Autodesk Inventor part; units mm, degrees
ref_plane "YZ Plane" through (0, 0, 0) normal (1, 0, 0) x (0, 1, 0)
ref_plane "XZ Plane" through (0, 0, 0) normal (0, 1, 0) x (-1, 0, 0)
ref_plane "XY Plane" through (0, 0, 0) normal (0, 0, 1) x (1, 0, 0)
sketch "Sketch1" plane through (0, 0, 0) normal (1, 0, 0) x (0, 1, 0)
  circle A0 centre (0, 0) radius 11
  circle A1 centre (0, 0) radius 22
  circle A2 centre (0, 0) radius 17.5
  circle A3 centre (17.5, 0) radius 2.75
  circle A4 centre (-8.75, 15.1554) radius 2.75
  circle A5 centre (-8.75, -15.1554) radius 2.75
  dimension "d2" = 35
  dimension "d0" = 22
  dimension "d1" = 44
  dimension "d3" = 5.5
  dimension "d6" = 360
extrude "Extrusion1" add sketch "Sketch1" along normal blind 7.5 contours A1 | A3 A2 A5 A4
sketch "Sketch2" plane through (7.5, 0, 0) normal (1, 0, 0) x (0, 0, -1)
  arc A0 (2.7415, 17.2839) -> (-2.7415, 17.2839) centre (0, 0) ccw
  circle A1 centre (0, 0) radius 17.5
  circle A2 centre (0, 17.5) radius 2.75
  circle A3 centre (-15.1554, -8.75) radius 2.75
  circle A4 centre (15.1554, -8.75) radius 2.75
  dimension "d10" = 35
  dimension "d11" = 5.5
  dimension "d14" = 360
extrude "Extrusion2" cut sketch "Sketch2" against normal blind 10 contours A2 A0 | A0 A2 | A3 A1 | A1 A3 | A4 A1 | A1 A4
sketch "Sketch3" plane through (7.5, 0, 0) normal (1, 0, 0) x (0, 0, -1)
  line L0 (0, 0) -> (0, -25)
  line L1 (0, 0) -> (25, 0) construction
  line L2 (0, -25) -> (50, -25)
  line L3 (0, -25) -> (25, -25)
  line L4 (25, -25) -> (25, -20)
  line L5 (25, -20) -> (0, -20)
  line L6 (0, -20) -> (0, -25)
  line L7 (0, -20) -> (30, -20)
  line L8 (30, -20) -> (30, -25)
  line L9 (30, -25) -> (0, -25)
  line L10 (0, -25) -> (0, -20)
  line L11 (30, -25) -> (-30, -25)
  line L12 (-30, -25) -> (-30, -20)
  line L13 (-30, -20) -> (30, -20)
  line L14 (30, -20) -> (30, -25)
  circle A0 centre (0, 0) radius 22
  line L15 (25, -25) -> (-22, -25)
  line L16 (-22, -25) -> (-22, 0)
  line L17 (-22, 0) -> (25, 0)
  line L18 (22, 0) -> (-22, 0)
  line L19 (-22, 0) -> (-22, -25)
  line L20 (-22, -25) -> (22, -25)
  line L21 (22, -25) -> (22, 0)
  line L22 (30, -20) -> (22, -20)
  line L23 (22, -20) -> (22, -25)
  line L24 (22, -25) -> (30, -25)
  line L25 (30, -25) -> (30, -20)
  line L26 (-30, -20) -> (-22, -20)
  line L27 (-22, -20) -> (-22, -25)
  line L28 (-22, -25) -> (-30, -25)
  line L29 (-30, -25) -> (-30, -20)
  dimension "d18" = 25
  dimension "d19" = 90
  dimension "d20" = 50
  dimension "d21" = 25
  dimension "d22" = 5
  dimension "d23" = 30
  dimension "d24" = 5
  dimension "d25" = 60
  dimension "d26" = 5
extrude "Extrusion3" add sketch "Sketch3" against normal blind 7.5 contours L5 A0 L0 | A0 L13 L16 | L21 L5 A0 | A0 L5 L21 L2 L0 | L0 L11 L16 L13 A0 | L16 L11 L12 L13 | L5 L4 L2 L21 | L7 L8 L2 L4
sketch "Sketch5" plane through (7.5, 0, 0) normal (1, 0, 0) x (0, 0, -1)
  line L0 (30, -20) -> (30, -25)
  line L1 (22, -20) -> (30, -20)
  line L2 (30, -25) -> (22, -25)
  line L3 (22, -25) -> (22, -20)
  line L4 (22, -20) -> (30, -20)
  line L5 (30, -20) -> (30, -25)
  line L6 (-30, -20) -> (-30, -25)
  line L7 (-30, -25) -> (-22, -25)
  line L8 (-22, -25) -> (-22, -20)
  line L9 (-22, -20) -> (-30, -20)
  line L10 (-30, -20) -> (-30, -25)
  point P0 (0, 0)
extrude "Extrusion5" add sketch "Sketch5" along normal blind 5
sketch "Sketch8" plane through (0, -20, 30) normal (0, 1, 0) x (1, 0, 0)
  circle A0 centre (3.125, 4) radius 1.5
  circle A1 centre (9.375, 4) radius 1.5
  circle A2 centre (9.375, 56) radius 1.5
  circle A3 centre (3.125, 56) radius 1.5
  point P0 (0, 8)
  point P1 (12.5, 0)
  point P2 (12.5, 52)
  point P3 (0, 60)
  point P4 (0, 52)
extrude "Extrusion7" cut sketch "Sketch8" against normal blind 5
properties part number "Slipring_mount"
Part model, mm, in its own coordinate system. A direction names the side the tool comes from. Give positions to 0.01 mm unless a question says otherwise; leave off trailing zeros. Loops run counter-clockwise (first coordinate to the right, second up) from the corner with the lowest first, then second, coordinate; pieces in that order, holes last. Notation, with made-up numbers: M -4.5,68.5 L 21.5,68.5 A12 cw 21.5,83.5 Z; hole C -5,77 d11. An arc over 180 degrees is marked long. Return JSON: item names as keys, results as strings.
1) Drill centre lines: line 1 (X direction, y = -21.65, z = -26) (3 decimals); line 2 (Z direction, x = 3.5, y = 0); line 3 (Z direction, x = 3.25, y = -7). Where is each one in solid material? Low to high.
Calculated:
{"line 1": "x = 0 to 1.625, 4.625 to 7.875, 10.875 to 12.5", "line 2": "z = -22 to -11, 11 to 22", "line 3": "z = -22 to -17.28, -13.03 to -8.49, 8.49 to 13.03, 17.28 to 22"}
2) Saw through at C-C, the plane x = 5.75. List the corners of the cut face in (y, z), then the cut area to 3 significant figures.
Calculated:
{"outline": "M -25,-30 L -20,-30 L -20,-22 L 0,-22 A22 ccw 0,22 L -20,22 L -20,30 L -25,30 Z; hole C -8.75,-15.16 d5.5; hole C -8.75,15.16 d5.5; hole C 0,0 d22; hole C 17.5,0 d5.5", "area": "1,490 mm2"}
3) Saw through at B-B, the plane y = -8.75. List the corners of the cut face in (x, z).
Calculated:
{"outline": "M 0,-22 L 7.5,-22 L 7.5,-17.91 L 0,-17.91 Z; M 0,-12.41 L 7.5,-12.41 L 7.5,-6.67 L 0,-6.67 Z; M 0,6.67 L 7.5,6.67 L 7.5,12.41 L 0,12.41 Z; M 0,17.91 L 7.5,17.91 L 7.5,22 L 0,22 Z"}
4) Saw through at D-D, the plane x = 3. List the corners of the cut face in (y, z), then the cut area to 3 significant figures.
Calculated:
{"outline": "M -25,-30 L -20,-30 L -20,-27.49 L -25,-27.49 Z; M -25,-24.51 L -20,-24.51 L -20,-22 L 0,-22 A22 ccw 0,22 L -20,22 L -20,24.51 L -25,24.51 Z; M -25,27.49 L -20,27.49 L -20,30 L -25,30 Z; hole C -8.75,-15.16 d5.5; hole C -8.75,15.16 d5.5; hole C 0,0 d22; hole C 17.5,0 d5.5", "area": "1,460 mm2"}
5) Saw through at A-A, the plane z = 26. List the corners of the cut face in (x, y) (3 decimals).
Calculated:
{"outline": "M 0,-25 L 1.625,-25 L 1.625,-20 L 0,-20 Z; M 4.625,-25 L 7.875,-25 L 7.875,-20 L 4.625,-20 Z; M 10.875,-25 L 12.5,-25 L 12.5,-20 L 10.875,-20 Z"}
6) 3-axis set-ups, long thin cutter, end or side, ignore diameter. For faces 4 (the face through (4, -10, -22)), 5 (the face through (4, 22, 0)), 6 (the face through (10, -23, -22)), 7 (the face through (4, -10, 22)): which of +Z, -Z, +X, -X, +Y, -Y reach the whole face in a straight line?
Calculated:
{"face 4": "-Z, +X, -X, +Y", "face 5": "+X, -X, +Y", "face 6": "+X, +Y, -Y", "face 7": "+Z, +X, -X, +Y"}
7) Flat gauge pins, fed straight in: pin 1 Ø4 at (x, y) = (7.5, 11) entering from +Z; pin 2 Ø1.5 at (x, y) = (2, 10.5) entering from +Z; pin 3 Ø1.5 at (x, y) = (3, -8) entering from -Z. Where does each tip first touch, or does it go through?
Calculated:
{"pin 1": "stops at z = 20.07", "pin 2": "stops at z = 19.72", "pin 3": "stops at z = -22"}
8) Pull direction X, two halves, no side cores. Call faces 1 (the face through (2.93, -22.465, 24.513)), 2 (the face through (0, -12, 0)), 3 (the face through (6, -23, 30)): released by +X, released by -X, zero draft, split by the parting line, or undercut.
Calculated:
{"face 1": "undercut", "face 2": "released by -X", "face 3": "zero draft"}
